Check sheet for the modelled part. Datum: model origin and axes. Units: mm. Give positions to 0.01 mm unless a question says otherwise; leave off trailing zeros. Loops run counter-clockwise (first coordinate to the right, second up) from the corner with the lowest first, then second, coordinate; pieces in that order, holes last. Notation, with made-up numbers: (81, 17) -> (118, 17) arc R24 ccw to (118, 50) -> close; hole circle Ø10 at (60.5, -35.5). An arc over 180 degrees is marked (long way). Write each question's results on one line, items separated by ' | '. Start each with the question number.
1. Cross-section at A-A on z = -67. Record the boundary of the cut face in (x, y), and give its area (3 significant figures).
2. Material ranges on L1, parallel to X at y = 0.5, z = -83; L2, parallel to X at y = 1, z = -12.5; L3, parallel to X at y = 2, z = -23, recorded low to high. Write a range as from..to.
3. Cross-section at B-B on x = -98. Record the boundary of the cut face in (y, z).
4. Cross-section at C-C on y = 3.5. Count the separate pieces of the cut face and the enclosed holes in it, and give its area (3 significant figures).
from build123d import *

# Parameters (mm, degrees)
SKETCH1_W           = 32
SKETCH1_H           = 6.1
SKETCH1_W_2         = 6.1
SKETCH1_H_2         = 20
SKETCH1_W_3         = 4
SKETCH1_H_3         = 10
BOSS_EXTRUDE1_DEPTH = 6.096


with BuildPart() as part:
    # Sketch1 → Boss-Extrude1 (new body)
    with BuildSketch(Plane(origin=(0, 0, 0), x_dir=(1, 0, 0), z_dir=(0, 1, 0))):
        with BuildLine():
            Line((-294.8, 100), (-10, 100))
            ThreePointArc((-10, 100), (-2.928932188, 97.071067812), (0, 90))
            Line((0, 90), (0, 10))
            ThreePointArc((0, 10), (-2.928932188, 2.928932188), (-10, 0))
            Line((-10, 0), (-294.8, 0))
            ThreePointArc((-294.8, 0), (-301.871067812, 2.928932188), (-304.8, 10))
            Line((-304.8, 10), (-304.8, 90))
            ThreePointArc((-304.8, 90), (-301.871067812, 97.071067812), (-294.8, 100))
        make_face()
        with Locations((-216.4, 86.95)):
            Rectangle(SKETCH1_W, SKETCH1_H, mode=Mode.SUBTRACT)
        with Locations((-152.4, 86.95)):
            Rectangle(SKETCH1_W, SKETCH1_H, mode=Mode.SUBTRACT)
        with Locations((-88.4, 86.95)):
            Rectangle(SKETCH1_W, SKETCH1_H, mode=Mode.SUBTRACT)
        with Locations((-219.35, 60)):
            Rectangle(SKETCH1_W_2, SKETCH1_H_2, mode=Mode.SUBTRACT)
        with Locations((-219.35, 20)):
            Rectangle(SKETCH1_W_2, SKETCH1_H_2, mode=Mode.SUBTRACT)
        with Locations((-27.4, 84.239115677)):
            Rectangle(SKETCH1_W_3, SKETCH1_H_3, mode=Mode.SUBTRACT)
        with Locations((-138.25, 60)):
            Rectangle(SKETCH1_W_2, SKETCH1_H_2, mode=Mode.SUBTRACT)
        with Locations((-138.25, 20)):
            Rectangle(SKETCH1_W_2, SKETCH1_H_2, mode=Mode.SUBTRACT)
        with Locations((-277.4, 80.703857292)):
            Rectangle(SKETCH1_W_3, SKETCH1_H_3, mode=Mode.SUBTRACT)
        with Locations((-92.15, 60)):
            Rectangle(SKETCH1_W_2, SKETCH1_H_2, mode=Mode.SUBTRACT)
        with Locations((-92.15, 20)):
            Rectangle(SKETCH1_W_2, SKETCH1_H_2, mode=Mode.SUBTRACT)
        with Locations((-277.4, 19.796375445)):
            Rectangle(SKETCH1_W_3, SKETCH1_H_3, mode=Mode.SUBTRACT)
        with Locations((-277.4, 51.677858863)):
            Rectangle(SKETCH1_W_3, SKETCH1_H_3, mode=Mode.SUBTRACT)
        with Locations((-27.4, 24.581782644)):
            Rectangle(SKETCH1_W_3, SKETCH1_H_3, mode=Mode.SUBTRACT)
        with Locations((-27.4, 55.358303889)):
            Rectangle(SKETCH1_W_3, SKETCH1_H_3, mode=Mode.SUBTRACT)
    extrude(amount=BOSS_EXTRUDE1_DEPTH)


solid = part.part
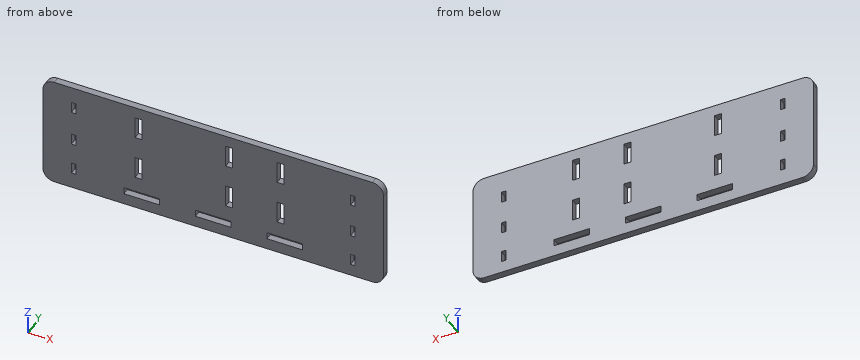
Geometry says:
1) outline: (-304.8, 0) -> (-222.4, 0) -> (-222.4, 6.1) -> (-304.8, 6.1) -> close; (-216.3, 0) -> (-141.3, 0) -> (-141.3, 6.1) -> (-216.3, 6.1) -> close; (-135.2, 0) -> (-95.2, 0) -> (-95.2, 6.1) -> (-135.2, 6.1) -> close; (-89.1, 0) -> (0, 0) -> (0, 6.1) -> (-89.1, 6.1) -> close | area: 1,750 mm^2
2) L1: -304.8..-279.4, -275.4..-29.4, -25.4..0 | L2: -304.8..-222.4, -216.3..-141.3, -135.2..-95.2, -89.1..0 | L3: -304.8..-279.4, -275.4..-222.4, -216.3..-141.3, -135.2..-95.2, -89.1..-29.4, -25.4..0
3) outline: (0, -100) -> (6.1, -100) -> (6.1, -90) -> (0, -90) -> close; (0, -83.9) -> (6.1, -83.9) -> (6.1, 0) -> (0, 0) -> close
4) separate pieces: 1 | enclosed holes: 15 | area: 28,800 mm^2
